Can you work these out from the drawing? Everything is in mm from the part's minimum corner. Round coordinates to 2 decimals unless told otherwise and drop trailing zeros. Write each loop counter-clockwise with the first axis right and the second up, starting at its lowest first coordinate (ties: lowest second). Pieces come first, ordered by that corner, then holes. Notation, with made-up numbers: (59, 84) -> (109, 84) arc R20 ccw to (109, 97) -> close; hole circle Ø7 at (5.25, 22.5). An arc over 180 degrees is marked (long way). Answer as CSV lines item,"result". Start each with the question number.
Q1. Imagine slicing it at C-C on z = 2.3. Please give me the cut outline in (x, y).
Q2. If I drill on line 1 (X direction, y = 12.75, z = 2.15); line 2 (Y direction, x = 69.5, z = 1.3); line 3 (X direction, y = 11.75, z = 2.65), over which ranges is the centre line in solid material (lowest first)? Write a range as [from, to].
Q3. Imagine slicing it at B-B on y = 12.5. Please give me the cut outline in (x, z).
Q4. Imagine slicing it at D-D on x = 44.5. Please give me the cut outline in (y, z).
Q5. Will these pins go through, and if not, where does the flat tip stop? pin 1 Ø3 at (x, y) = (43.5, 9.5) entering from -Z; pin 2 Ø1.5 at (x, z) = (8.5, 1) entering from -Y; pin 3 Ø1 at (x, z) = (14, 1) entering from -Y.
Q6. Imagine slicing it at A-A on x = 12.5. Please give me the cut outline in (y, z).
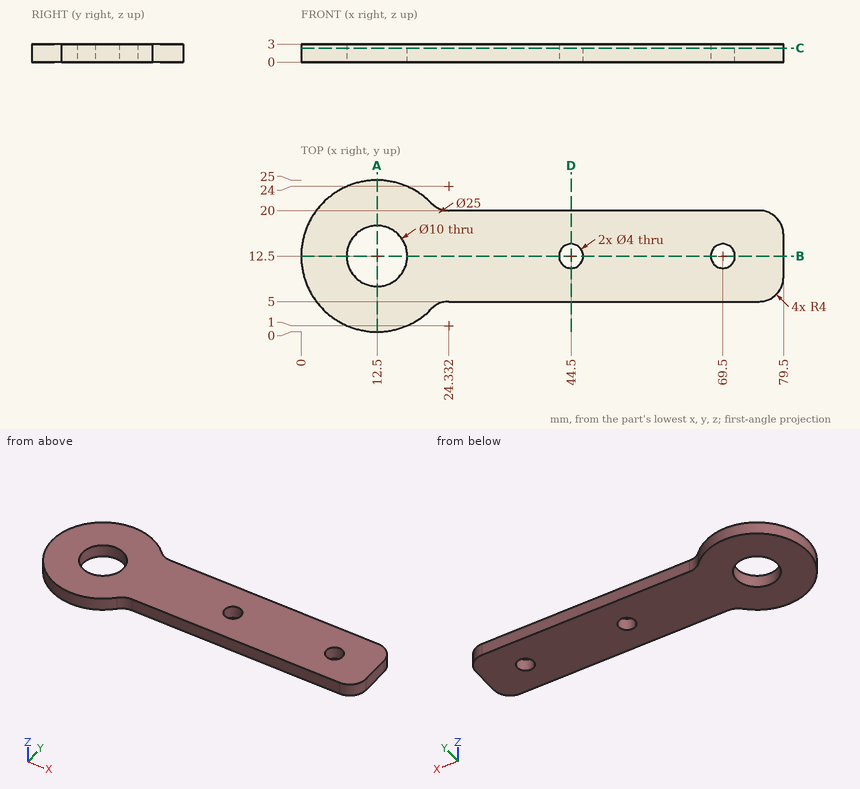
Checks:
1,outline,"(21.46, 3.79) arc R4 cw to (24.33, 5) -> (75.5, 5) arc R4 ccw to (79.5, 9) -> (79.5, 16) arc R4 ccw to (75.5, 20) -> (24.33, 20) arc R4 cw to (21.46, 21.21) arc R12.5 ccw (long way) to start; hole circle Ø10 at (12.5, 12.5); hole circle Ø4 at (44.5, 12.5); hole circle Ø4 at (69.5, 12.5)"
2,line 1,"[0, 7.51], [17.49, 42.52], [46.48, 67.52], [71.48, 79.5]"
2,line 2,"[5, 10.5], [14.5, 20]"
2,line 3,"[0.02, 7.56], [17.44, 42.65], [46.35, 67.65], [71.35, 79.5]"
3,outline,"(0, 0) -> (7.5, 0) -> (7.5, 3) -> (0, 3) -> close; (17.5, 0) -> (42.5, 0) -> (42.5, 3) -> (17.5, 3) -> close; (46.5, 0) -> (67.5, 0) -> (67.5, 3) -> (46.5, 3) -> close; (71.5, 0) -> (79.5, 0) -> (79.5, 3) -> (71.5, 3) -> close"
4,outline,"(5, 0) -> (10.5, 0) -> (10.5, 3) -> (5, 3) -> close; (14.5, 0) -> (20, 0) -> (20, 3) -> (14.5, 3) -> close"
5,pin 1,"z = 0"
5,pin 2,"y = 0.43"
5,pin 3,"y = 0.04"
6,outline,"(0, 0) -> (7.5, 0) -> (7.5, 3) -> (0, 3) -> close; (17.5, 0) -> (25, 0) -> (25, 3) -> (17.5, 3) -> close"
